Geometry: final body of the model. Coordinates: model frame, mm. Face numbers are marked on the shaded views. Give positions to 0.01 mm unless a question says otherwise; leave off trailing zeros. Write each loop counter-clockwise with the first axis right and the second up, starting at its lowest first coordinate (ties: lowest second). Pieces come first, ordered by that corner, then holes.
Q1. Pin query (flat end, axial travel): pin 1 (12 mm diameter, centred on x = -24.5, y = 17.5, fed in from +Z); pin 2 (1.5 mm diameter, centred on x = 7.5, y = 2.5, fed in from -Z); pin 3 (6 mm diameter, centred on y = 3, z = 3, fed in from -X) (3 decimals); pin 4 (8 mm diameter, centred on x = 6.5, z = 14, fed in from +Y). Return the tip coordinate at first contact, or that it passes through.
Q2. Line query: L1, parallel to Y at x = -29.21, z = -6.45; L2, parallel to X at y = 7, z = 0 (3 decimals); L3, parallel to X at y = 20.5, z = 10.5. Output: solid intervals per line, ascending.
Q3. Cut plane C-C on y = 12.7. Count the separate pieces of the cut face and the enclosed holes in it, plus the area to 3 significant figures.
Q4. Cut plane B-B on z = 0. Return the cut outline in (x, y) (3 decimals), plus the area to 3 significant figures.
Q5. Draft query along X for the marked faces 1 and 2. Return one class per face: pulls with the +X half, pulls with the -X half, needs draft (parallel to the pull), parting line crosses it, or undercut.
Q6. Cut plane A-A on x = 29.21. Return the cut outline in (y, z).
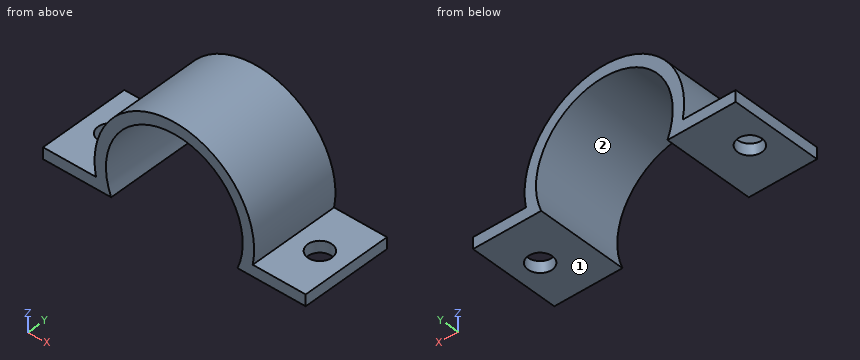
```python
from build123d import *

# Parameters (mm, degrees)
SKETCH1_R           = 19.05
BOSS_EXTRUDE1_DEPTH = 25.4
SKETCH2_R           = 3.3782
CUT_EXTRUDE1_DEPTH  = 36.8775
SKETCH3_W           = 84.126846883
SKETCH3_H           = 24.140829336
CUT_EXTRUDE2_DEPTH  = 26.4


with BuildPart() as part:
    # Sketch1 → Boss-Extrude1 (new body)
    with BuildSketch(Plane(origin=(0, 0, 0), x_dir=(1, 0, 0), z_dir=(0, 1, 0))):
        with BuildLine():
            Line((36.587384889, 13.6525), (17.537384889, 13.6525))
            ThreePointArc((17.537384889, 13.6525), (0, 22.225), (-17.537384889, 13.6525))
            Line((-17.537384889, 13.6525), (-36.587384889, 13.6525))
            Line((-36.587384889, 13.6525), (-36.587384889, 4.1275))
            Line((-36.587384889, 4.1275), (-21.838369187, 4.1275))
            ThreePointArc((-21.838369187, 4.1275), (0, -22.225), (21.838369187, 4.1275))
            Line((21.838369187, 4.1275), (36.587384889, 4.1275))
            Line((36.587384889, 4.1275), (36.587384889, 13.6525))
        make_face()
        Circle(SKETCH1_R, mode=Mode.SUBTRACT)
    extrude(amount=BOSS_EXTRUDE1_DEPTH)

    # Sketch2 → Cut-Extrude1 (cut, through all)
    with BuildSketch(Plane(origin=(0, 0, -13.6525), x_dir=(-1, 0, 0), z_dir=(0, 0, -1))):
        with Locations((29.21, 12.7)):
            Circle(SKETCH2_R)
        with Locations((-29.21, 12.7)):
            Circle(SKETCH2_R)
    extrude(amount=-CUT_EXTRUDE1_DEPTH, mode=Mode.SUBTRACT)

    # Sketch3 → Cut-Extrude2 (cut, through all)
    with BuildSketch(Plane(origin=(0, 25.4, 0), x_dir=(1, 0, 0), z_dir=(0, 1, 0))):
        with Locations((0.41143502, 19.372914668)):
            Rectangle(SKETCH3_W, SKETCH3_H)
    extrude(amount=-CUT_EXTRUDE2_DEPTH, mode=Mode.SUBTRACT)


solid = part.part
```
Data:
1. pin 1: stops at z = 12.32
1. pin 2: stops at z = 17.17
1. pin 3: stops at x = -22.225
1. pin 4: stops at y = 25.4
2. L1: y = 0 to 9.32, 16.08 to 25.4
2. L2: x = -22.225 to -19.05, 19.05 to 22.225
2. L3: x = -19.59 to -15.9, 15.9 to 19.59
3. separate pieces: 3
3. enclosed holes: 0
3. area: 306 mm2
4. outline: (-22.225, 0) - (-19.05, 0) - (-19.05, 25.4) - (-22.225, 25.4) - close; (19.05, 0) - (22.225, 0) - (22.225, 25.4) - (19.05, 25.4) - close
4. area: 161 mm2
5. face 1: needs draft
5. face 2: undercut
6. outline: (0, -7.3) - (9.32, -7.3) - (9.32, -4.13) - (0, -4.13) - close; (16.08, -7.3) - (25.4, -7.3) - (25.4, -4.13) - (16.08, -4.13) - close
